Part model, mm, in its own coordinate system. A direction names the side the tool comes from. Coordinates: 2 decimals unless noted, no trailing zeros. Loops run counter-clockwise (first coordinate to the right, second up) from the corner with the lowest first, then second, coordinate; pieces in that order, holes last. Notation, with made-up numbers: (38, -37.75) -> (79, -37.75) arc R22 cw to (79, -22.75) -> close; hole circle Ø9 at (27.5, 40.25). An arc over 180 degrees is marked (long way). Use one line per item in the form item = value. Start each with the question number.
(1) Band-saw the part on C-C on x = 26. Give the cut face in (y, z), then the cut area to 3 significant figures.
(2) Pin check, flat tips, straight feed: P1, Ø6, axis at x = 0.5, z = -12, coming from the +Y side; P2, Ø0.6, axis at y = 0.5, z = 21.5, coming from the +X side; P3, Ø5.5, axis at x = 54.3, z = 50.97, coming from the -Y side; P4, Ø4.5, axis at x = 30.92, z = 7.67, coming from the +Y side. Stop position of each tip, or through.
(3) Mould opens along X. For faces 3 (the flat face through (44.906, 9, 1)), 4 (the flat face through (13, 0, 31)), 5 (the cylindrical face through (-11.44, 3.014, 48.242)), 6 (the cylindrical face through (11.943, 3.014, 48.242)) say: +X half, -X half, draft (parallel to the pull), parting line (faces both ways), or undercut.
(4) Band-saw the part on B-B on z = 14.5. Give the cut face in (x, y).
(5) Band-saw the part on A-A on y = 8.75. Give the cut face in (x, z).
(6) 3-axis set-ups, long thin cutter, end or side, ignore diameter. For faces 1 (the cylindrical face through (0.837, 0.986, 28.984)), 2 (the cylindrical face through (39.68, 7.94, 0.27)): which of +Z, -Z, +X, -X, +Y, -Y reach the whole face in a straight line?
(7) Band-saw the part on D-D on x = 7.5. Give the cut face in (y, z), then the cut area to 3 significant figures.
(8) Drill centre lines: L1, parallel to X at y = 8, z = -1.5; L2, parallel to Z at x = -9, y = 2.75; L3, parallel to X at y = 1.25, z = -5. Where is each one in solid material? Low to high. Write a range as [from, to].
```python
from build123d import *

# Parameters (mm, degrees)
SKETCH_1_W                   = 18.5
SKETCH_1_H                   = 4
HOLE_WIZARD_M3_1_D           = 3.5
HOLE_WIZARD_M3_1_CBORE_D     = 5.5
HOLE_WIZARD_M3_1_CBORE_DEPTH = 2
SKETCH_9_R                   = 4.078764036
EXTRUDE_2_DEPTH              = 4
SKETCH_10_R                  = 3
EXTRUDE_3_DEPTH              = 8
CUT_EXTRUDE_START            = -6.5
CUT_EXTRUDE_2_DEPTH          = 6.5
PATTERN_CIRCULAR_1_COUNT     = 3
PATTERN_CIRCULAR_1_ANGLE     = 120
SKETCH_13_W                  = 2.125984269
SKETCH_13_H                  = 7.532431529
EXTRUDE_4_DEPTH              = 0.8
SKETCH_14_W                  = 7.649512524
SKETCH_14_H                  = 1.311345004
SKETCH_14_H_2                = 1.033306543
EXTRUDE_5_DEPTH              = 0.8


with BuildPart() as part:
    # Sketch 1 → Revolve 1 (revolve)
    with BuildSketch(Plane.XY.offset(0.922906258), mode=Mode.PRIVATE) as revolve_1_sk:
        with Locations((9.859359688, 2)):
            Rectangle(SKETCH_1_W, SKETCH_1_H)
    revolve(revolve_1_sk.sketch.rotate(Axis((0.609359688, 4, 0.922906258), (0, -1, 0)), 270), axis=Axis((0.609359688, 4, 0.922906258), (0, -1, 0)))

    # Hole Wizard M3 _1 (through all)
    with Locations(Plane(origin=(0, 4, 0), x_dir=(1, 0, 0), z_dir=(0, 1, 0))):
        with Locations((-11.081983263, -7.672906258), (12.300702639, -7.672906258), (0.609359688, 12.577093742)):
            hole_wizard_m3_1 = CounterBoreHole(HOLE_WIZARD_M3_1_D / 2, HOLE_WIZARD_M3_1_CBORE_D / 2, HOLE_WIZARD_M3_1_CBORE_DEPTH)

    # Sketch 9 → Extrude 2 (add)
    with BuildSketch(Plane.XZ):
        with Locations((0.609359688, 0.922906258)):
            Circle(SKETCH_9_R)
    extrude(amount=-EXTRUDE_2_DEPTH)

    # Sketch 10 → Extrude 3 (add)
    with BuildSketch(Plane(origin=(0, 4, 0), x_dir=(1, 0, 0), z_dir=(0, 1, 0))):
        with Locations(Location((0.609359688, -0.922906258, 0), (0, 0, 270))):
            Circle(SKETCH_10_R)
    extrude(amount=EXTRUDE_3_DEPTH)

    # Sketch 11 → Cut-Extrude 2 (cut)
    with BuildSketch(Plane(origin=(0, 12, 0), x_dir=(1, 0, 0), z_dir=(0, 1, 0)).offset(CUT_EXTRUDE_START)):
        with BuildLine():
            Line((2.905866026, 1.007393885), (2.905866026, -2.853206401))
            ThreePointArc((2.905866026, -2.853206401), (3.609359688, -0.922906258), (2.905866026, 1.007393885))
        make_face()
    extrude(amount=CUT_EXTRUDE_2_DEPTH, mode=Mode.SUBTRACT)

    # Pattern Circular 1: Hole Wizard M3 _1 ×3 about axis
    pattern_circular_1_axis = Axis((0.609359688, 0, 0.922906258), (0, -1, 0))
    for i in range(1, PATTERN_CIRCULAR_1_COUNT):
        add(hole_wizard_m3_1.rotate(pattern_circular_1_axis, i * PATTERN_CIRCULAR_1_ANGLE / (PATTERN_CIRCULAR_1_COUNT - 1)), mode=Mode.SUBTRACT)


with BuildPart() as body_2:
    # Move Body 3: copy of part
    add(part.part.moved(Location((0, 0, 43.295994543))))


with BuildPart() as part_1:
    add(part.part)

    add(body_2.part)  # Extrude 4 merges body 2
    # Sketch 13 → Extrude 4 (add)
    with BuildSketch(Plane.XZ):
        with Locations((-0.453632447, 22.075248032)):
            Rectangle(SKETCH_13_W, SKETCH_13_H)
    extrude(amount=-EXTRUDE_4_DEPTH)


with BuildPart() as body_2_2:
    # Move Body 4: copy of part
    add(part_1.part.moved(Location((42, 0, 0))))


with BuildPart() as part_2:
    add(part_1.part)

    add(body_2_2.part)  # Extrude 5 merges body 2 2
    # Sketch 14 → Extrude 5 (add)
    with BuildSketch(Plane.XZ):
        with Locations((21.609359688, 44.317374847)):
            Rectangle(SKETCH_14_W, SKETCH_14_H)
        with Locations((21.609359688, -0.516653272)):
            Rectangle(SKETCH_14_W, SKETCH_14_H_2)
    extrude(amount=-EXTRUDE_5_DEPTH)


solid = part_2.part
```
A:
q1.outline = (0, -7.22) -> (4, -7.22) -> (4, 9.07) -> (0, 9.07) -> close; (0, 36.07) -> (4, 36.07) -> (4, 52.37) -> (0, 52.37) -> close
q1.area = 130 mm²
q2.P1 = 4
q2.P2 = 42.61
q2.P3 = 0
q2.P4 = 2
q3.face_3 = +X half
q3.face_4 = draft
q3.face_5 = undercut
q3.face_6 = undercut
q4.outline = (-11.96, 0) -> (-1.14, 0) -> (-1.14, 2) -> (-2.14, 2) -> (-2.14, 4) -> (-11.96, 4) -> close; (2.36, 0) -> (13.18, 0) -> (13.18, 4) -> (3.36, 4) -> (3.36, 2) -> (2.36, 2) -> close; (30.04, 0) -> (40.86, 0) -> (40.86, 2) -> (39.86, 2) -> (39.86, 4) -> (30.04, 4) -> close; (44.36, 0) -> (55.18, 0) -> (55.18, 4) -> (45.36, 4) -> (45.36, 2) -> (44.36, 2) -> close
q5.outline = (2.91, -1.01) -> (2.91, 2.85) arc R3 ccw (long way) to start; (2.91, 42.29) -> (2.91, 46.15) arc R3 ccw (long way) to start; (44.91, -1.01) -> (44.91, 2.85) arc R3 ccw (long way) to start; (44.91, 42.29) -> (44.91, 46.15) arc R3 ccw (long way) to start
q6.face_1 = +Y, -Y
q6.face_2 = +Y
q7.outline = (0, -16.25) -> (4, -16.25) -> (4, 18.09) -> (0, 18.09) -> close; (0, 27.05) -> (4, 27.05) -> (4, 61.39) -> (0, 61.39) -> close
q7.area = 275 mm²
q8.L1 = [-1.16, 2.38], [40.84, 44.38]
q8.L2 = [-14.89, -7.62], [-4.03, 5.88], [9.47, 16.73], [28.41, 35.67], [39.27, 49.17], [52.77, 60.03]
q8.L3 = [-16.92, -12.62], [-9.54, 10.76], [13.84, 18.14], [25.08, 29.38], [32.46, 52.76], [55.84, 60.14]
